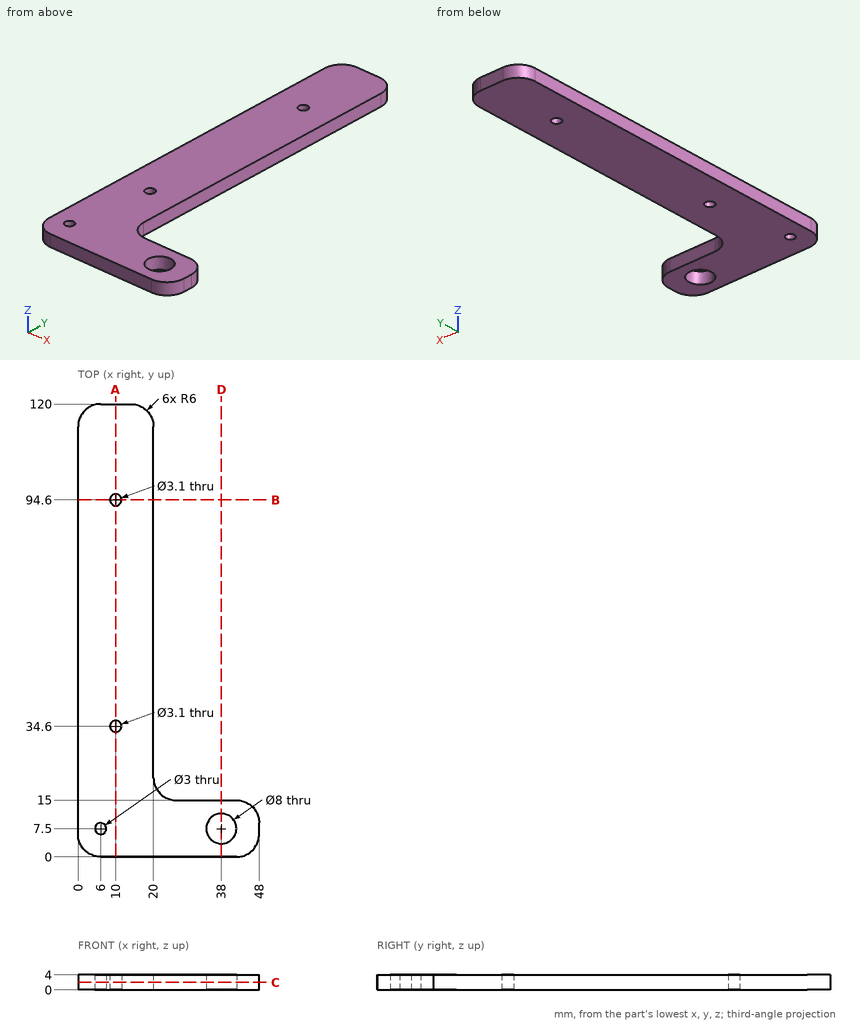
Design review of the part shown in the three views and the two pictorial views. Dimensions are in mm from the part's minimum x, y and z. Coordinates: 2 decimals unless noted, no trailing zeros. Loops run counter-clockwise (first coordinate to the right, second up) from the corner with the lowest first, then second, coordinate; pieces in that order, holes last. Notation, with made-up numbers: (79, 32) - (94, 32) arc R12 cw to (94, 43) - close; hole circle Ø9 at (69, 33.5). An arc over 180 degrees is marked (long way). Use a Markdown table: item, result. Add a question column.
Item 1: We need section C-C (z = 2). Give the boundary of the cut face in (x, y), and give its area (3 significant figures).
Item 2: We need section D-D (x = 38). Give the boundary of the cut face in (y, z), and give its area (3 significant figures).
Item 3: We need section B-B (y = 94.6). Give the boundary of the cut face in (x, z), and give its area (3 significant figures).
Item 4: For line 1 (Y direction, x = 10, z = 3.3); line 2 (Y direction, x = 38, z = 1.4); line 3 (X direction, y = 94.6, z = 1.5), list the stretches that pass through material, from the lowest coordinate up.
Item 5: We need section A-A (x = 10). Give the boundary of the cut face in (y, z), and give its area (3 significant figures).
Item 6: Insertion check: pin 1 Ø4 at (x, y) = (10, 94.6) entering from -Z; pin 2 Ø2 at (x, z) = (32, 2.5) entering from +Y; pin 3 Ø2 at (y, z) = (70.5, 2) entering from +X. Each pin has a flat end and moves straight along its axis. Give the tip position at first contact, or say it passes through.
Results list:
| question | item | result |
|---|---|---|
| 1 | outline | (0, 6) arc R6 ccw to (6, 0) - (42, 0) arc R6 ccw to (48, 6) - (48, 9) arc R6 ccw to (42, 15) - (26, 15) arc R6 cw to (20, 21) - (20, 114) arc R6 ccw to (14, 120) - (6, 120) arc R6 ccw to (0, 114) - close; hole circle Ø3 at (6, 7.5); hole circle Ø3.1 at (10, 34.6); hole circle Ø3.1 at (10, 94.6); hole circle Ø8 at (38, 7.5) |
| 1 | area | 2,720 mm^2 |
| 2 | outline | (0, 0) - (3.5, 0) - (3.5, 4) - (0, 4) - close; (11.5, 0) - (15, 0) - (15, 4) - (11.5, 4) - close |
| 2 | area | 28.0 mm^2 |
| 3 | outline | (0, 0) - (8.45, 0) - (8.45, 4) - (0, 4) - close; (11.55, 0) - (20, 0) - (20, 4) - (11.55, 4) - close |
| 3 | area | 67.6 mm^2 |
| 4 | line 1 | y = 0 to 33.05, 36.15 to 93.05, 96.15 to 120 |
| 4 | line 2 | y = 0 to 3.5, 11.5 to 15 |
| 4 | line 3 | x = 0 to 8.45, 11.55 to 20 |
| 5 | outline | (0, 0) - (33.05, 0) - (33.05, 4) - (0, 4) - close; (36.15, 0) - (93.05, 0) - (93.05, 4) - (36.15, 4) - close; (96.15, 0) - (120, 0) - (120, 4) - (96.15, 4) - close |
| 5 | area | 455 mm^2 |
| 6 | pin 1 | stops at z = 0 |
| 6 | pin 2 | stops at y = 15 |
| 6 | pin 3 | stops at x = 20 |
